Input: part model. Units: mm. Frame: model coordinates. A direction names the side the tool comes from. Coordinates: 2 decimals unless noted, no trailing zeros. Loops run counter-clockwise (first coordinate to the right, second up) from the corner with the lowest first, then second, coordinate; pieces in that order, holes last. Notation, with made-up numbers: (53, 4.5) - (90, 4.5) arc R22 ccw to (90, 20.5) - close; hole circle Ø2 at (4.25, 68.5). An arc over 180 degrees is marked (long way). Use a Markdown table: item, result. Add a question column.
1. Section query C-C on z = 39. Return the cut outline in (x, y) (3 decimals).
2. Draft query along Z for faces 4 (the face through (-39, -1.588, 75)), 5 (the face through (40, -2, 79)), 6 (the face through (-40, -2, -79)). Return one class per face: released by +Z, released by -Z, zero draft, split by the parting line, or undercut.
3. Access query for faces 1 (the face through (-31.027, -2.103, 63.553)), 2 (the face through (1, -1, 1)), 3 (the face through (40.5, -2, 61)). Directions: +Z, -Z, +X, -X, +Y, -Y. A direction counts if a zero-diameter tool reaches every point of the face in a straight line with its end or side. Return the directions, or none.
4. Section query D-D on x = -26. Return the cut outline in (y, z) (3 decimals), then the cut area to 3 significant figures.
5. Section query A-A on z = -48.5. Return the cut outline in (x, y) (3 decimals).
6. Section query B-B on x = -0.5. Return the cut outline in (y, z) (3 decimals), then the cut area to 3 significant figures.
7. Contact query for flat-ended pins moving along their axis: P1, Ø1.8, axis at x = 40.24, z = 76.24, coming from the -Y side; P2, Ø1.6, axis at x = -11.5, y = -2, coming from the +Z side; P3, Ø6.5, axis at x = 40.24, z = 76.24, coming from the -Y side (3 decimals); P4, Ø1.7, axis at y = -2, z = 42.5, coming from the -X side. Output: stop coordinate, or through.
8. Ray query, L1, parallel to X at y = -2.5, z = -15.5; L2, parallel to X at y = -2.2, z = 4.5; L3, parallel to X at y = -2.85, z = 51. Return the intervals inside material, ascending. Write a range as [from, to].
```python
from build123d import *

# Parameters (mm, degrees)
F1_R      = 1.5
F1_W      = 24
F1_H      = 4
F2_DEPTH  = 3.175
F3_SIZE   = 2.49999
F4_R      = 1
F5_R      = 2.5
F6_DEPTH  = 1.5875
F7_W      = 15
F7_H      = 57
F7_W_2    = 30
F7_H_2    = 8
F8_DEPTH  = 3.176
F9_SIZE   = 1.5
F10_SIZE  = 1.5
F11_R     = 1
F12_W     = 78.25
F12_H     = 150.25
F13_DEPTH = 1


# Not quite as in the source:
# - a fillet or chamfer is up to 0.001 mm smaller than in the source, because OpenCascade refuses the exact size


with BuildPart() as f2:
    # F1 (on Front) → F2 (new body)
    with BuildSketch(Plane.XZ):
        Polygon((43, 73.2426406871), (43, 79), (37.2426406871, 79), (37.2426406871, 76.5), (-37.2426406871, 76.5), (-37.2426406871, 79), (-43, 79), (-43, 73.2426406871), (-40.5, 73.2426406871), (-40.5, -73.2426406871), (-43, -73.2426406871), (-43, -79), (-37.2426406871, -79), (-37.2426406871, -76.5), (-5, -76.5), (-5, -75), (5, -75), (5, -76.5), (37.2426406871, -76.5), (37.2426406871, -79), (43, -79), (43, -73.2426406871), (40.5, -73.2426406871), (40.5, 0), (39, 0), (39, 50), (40.5, 50), (40.5, 73.2426406871), align=None)
        with Locations((-40.2426406871, -76.2426406871)):
            Circle(F1_R, mode=Mode.SUBTRACT)
        with Locations((0, -61)):
            Rectangle(F1_W, F1_H, mode=Mode.SUBTRACT)
        with Locations((40.2426406871, -76.2426406871)):
            Circle(F1_R, mode=Mode.SUBTRACT)
        with Locations((-40.2426406871, 76.2426406871)):
            Circle(F1_R, mode=Mode.SUBTRACT)
        with BuildLine():
            ThreePointArc((-7.5, 58.5), (0, 66), (7.5, 58.5))
            Line((7.5, 58.5), (7.5, 25.5))
            ThreePointArc((7.5, 25.5), (0, 18), (-7.5, 25.5))
            Line((-7.5, 25.5), (-7.5, 58.5))
        make_face(mode=Mode.SUBTRACT)
        with Locations((40.2426406871, 76.2426406871)):
            Circle(F1_R, mode=Mode.SUBTRACT)
    extrude(amount=F2_DEPTH)

    # F3 (size 2.5 in the source; OpenCascade refuses exactly that, so slightly less here)
    f3_edges = [f2.edges().sort_by_distance(p)[0] for p in [
        (-37.242641, -1.5875, 76.5),
        (-40.5, -1.5875, 73.242641),
        (37.242641, -1.5875, 76.5),
        (40.5, -1.5875, 73.242641),
        (40.5, -1.5875, -73.242641),
        (37.242641, -1.5875, -76.5),
        (-37.242641, -1.5875, -76.5),
        (-40.5, -1.5875, -73.242641),
    ]]
    chamfer(f3_edges, length=F3_SIZE)

    # F4
    f4_edges = [f2.edges().sort_by_distance(p)[0] for p in [
        (43, -1.5875, 79),
        (-43, -1.5875, 79),
        (43, -1.5875, -79),
        (-43, -1.5875, -79),
        (40.5, -1.5875, 50),
        (40.5, -1.5875, 0),
    ]]
    fillet(f4_edges, radius=F4_R)

    # F5 (on face) → F6 (cut)
    with BuildSketch(Plane.XZ.offset(3.175)):
        with Locations((-40.2426406871, 76.2426406871)):
            Circle(F5_R)
        with Locations((40.2426406871, 76.2426406871)):
            Circle(F5_R)
        with Locations((40.2426406871, -76.2426406871)):
            Circle(F5_R)
        with Locations((-40.2426406871, -76.2426406871)):
            Circle(F5_R)
    extrude(amount=-F6_DEPTH, mode=Mode.SUBTRACT)

    # F7 (on face) → F8 (cut, through all)
    with BuildSketch(Plane.XZ.offset(3.175)):
        Polygon((-20.5, -66.5), (-20.5, 66.5), (-34.5, 70.5), (-28.5, 58.5), (-28.5, -58.5), (-34.5, -70.5), align=None)
        Polygon((34.5, 70.5), (20.5, 66.5), (20.5, -66.5), (34.5, -70.5), (28.5, -58.5), (28.5, 58.5), align=None)
        with Locations((0, 42)):
            Rectangle(F7_W, F7_H)
        with Locations((0, -61)):
            Rectangle(F7_W_2, F7_H_2)
    extrude(amount=-F8_DEPTH, mode=Mode.SUBTRACT)

    # F9
    f9_edges = [f2.edges().sort_by_distance(p)[0] for p in [
        (7.5, -1.5875, 70.5),
        (-7.5, -1.5875, 70.5),
        (-7.5, -1.5875, 13.5),
        (7.5, -1.5875, 13.5),
    ]]
    chamfer(f9_edges, length=F9_SIZE)

    # F10
    f10_edges = [f2.edges().sort_by_distance(p)[0] for p in [
        (-15, -1.5875, -65),
        (-15, -1.5875, -57),
        (15, -1.5875, -57),
        (15, -1.5875, -65),
    ]]
    chamfer(f10_edges, length=F10_SIZE)

    # F11
    f11_edges = [f2.edges().sort_by_distance(p)[0] for p in [
        (-34.5, -1.5875, 70.5),
        (-20.5, -1.5875, 66.5),
        (20.5, -1.5875, 66.5),
        (34.5, -1.5875, 70.5),
        (34.5, -1.5875, -70.5),
        (20.5, -1.5875, -66.5),
        (-34.5, -1.5875, -70.5),
        (-20.5, -1.5875, -66.5),
    ]]
    fillet(f11_edges, radius=F11_R)

    # F12 (on face) → F13 (cut)
    with BuildSketch(Plane(origin=(0, 0, 0), x_dir=(-1, 0, 0), z_dir=(0, 1, 0))):
        Rectangle(F12_W, F12_H)
    extrude(amount=-F13_DEPTH, mode=Mode.SUBTRACT)


solid = f2.part
```
Resolved:
| question | item | result |
|---|---|---|
| 1 | outline | (-40.5, -3.175) - (-28.5, -3.175) - (-28.5, -1) - (-39.125, -1) - (-39.125, 0) - (-40.5, 0) - close; (-20.5, -3.175) - (-7.5, -3.175) - (-7.5, -1) - (-20.5, -1) - close; (7.5, -3.175) - (20.5, -3.175) - (20.5, -1) - (7.5, -1) - close; (28.5, -3.175) - (39, -3.175) - (39, -1) - (28.5, -1) - close |
| 2 | face 4 | undercut |
| 2 | face 5 | released by +Z |
| 2 | face 6 | released by -Z |
| 3 | face 1 | +Y, -Y |
| 3 | face 2 | +Y |
| 3 | face 3 | +X, +Y, -Y |
| 4 | outline | (-3.175, -76.5) - (0, -76.5) - (0, -75.125) - (-1, -75.125) - (-1, -68.071) - (-3.175, -68.071) - close; (-3.175, 68.071) - (-1, 68.071) - (-1, 75.125) - (0, 75.125) - (0, 76.5) - (-3.175, 76.5) - close |
| 4 | area | 39.4 mm² |
| 5 | outline | (-40.5, -3.175) - (-28.5, -3.175) - (-28.5, -1) - (-39.125, -1) - (-39.125, 0) - (-40.5, 0) - close; (-20.5, -3.175) - (20.5, -3.175) - (20.5, -1) - (-20.5, -1) - close; (28.5, -3.175) - (40.5, -3.175) - (40.5, 0) - (39.125, 0) - (39.125, -1) - (28.5, -1) - close |
| 6 | outline | (-3.175, -75) - (-1, -75) - (-1, -65) - (-3.175, -65) - close; (-3.175, -57) - (-1, -57) - (-1, 13.5) - (-3.175, 13.5) - close; (-3.175, 70.5) - (-1, 70.5) - (-1, 75.125) - (0, 75.125) - (0, 76.5) - (-3.175, 76.5) - close |
| 6 | area | 190 mm² |
| 7 | P1 | through |
| 7 | P2 | z = 76.5 |
| 7 | P3 | y = -3.175 |
| 7 | P4 | x = -40.5 |
| 8 | L1 | [-40.5, -28.5], [-20.5, 20.5], [28.5, 40.5] |
| 8 | L2 | [-40.5, -28.5], [-20.5, 20.5], [28.5, 39] |
| 8 | L3 | [-40.5, -28.5], [-20.5, -7.5], [7.5, 20.5], [28.5, 40.5] |
